```python
from build123d import *

# Parameters (mm, degrees)
F0_W     = 38.1
F0_H     = 50.8
F1_DEPTH = 18.288
F2_SIZE  = 5.08


with BuildPart() as f1:
    # F0 (on Top) → F1 (new body)
    with BuildSketch(Plane.XY):
        with Locations((32.766, -53.848)):
            Rectangle(F0_W, F0_H)
        Polygon((65.532, -18.288), (0, -18.288), (0, 0), (-1.016, 0), (-4.572, -18.288), (-4.572, -28.448), (13.716, -28.448), (51.816, -28.448), (70.104, -28.448), (70.104, -18.288), (66.548, 0), (65.532, 0), align=None)
    extrude(amount=F1_DEPTH)

    # F2
    f2_edges = [f1.edges().sort_by_distance(p)[0] for p in [
        (13.716, -53.848, 18.288),
        (51.816, -53.848, 18.288),
        (51.816, -53.848, 0),
        (13.716, -53.848, 0),
        (-4.572, -28.448, 9.144),
        (70.104, -28.448, 9.144),
    ]]
    chamfer(f2_edges, length=F2_SIZE)


solid = f1.part
```
The listing builds one solid part. Answer for the finished solid, in the listing's coordinates (mm). A direction names the side the tool comes from. Give positions to 0.01 mm unless a question says otherwise; leave off trailing zeros. Order: outer loops, then holes, each group sorted by start corner. A loop starts at its lowest first (then second) coordinate and runs counter-clockwise, first axis right, second up. Notation, with made-up numbers: (-35, -2) -> (2, -2) arc R11 cw to (2, 7) -> close; hole circle Ø10 at (15.25, 78.5). An arc over 180 degrees is marked (long way). One line per item, written item: value.
1) Find section C-C, the plane y = -11.5. Determine the outline of the cut face in (x, z), plus the area to 3 significant figures.
Reported:
outline: (-3.25, 0) -> (0, 0) -> (0, 18.29) -> (-3.25, 18.29) -> close; (65.53, 0) -> (68.78, 0) -> (68.78, 18.29) -> (65.53, 18.29) -> close
area: 119 mm^2
2) Find section A-A, the plane y = -53. Determine the outline of the cut face in (x, z), plus the area to 3 significant figures.
Reported:
outline: (13.72, 5.08) -> (18.8, 0) -> (46.74, 0) -> (51.82, 5.08) -> (51.82, 13.21) -> (46.74, 18.29) -> (18.8, 18.29) -> (13.72, 13.21) -> close
area: 645 mm^2
3) A tool of negligible diameter and unlimited length cuts with its end or side. For faces 4 (the flat face through (49.24, -54.204, 15.784)), 5 (the flat face through (33, -18.288, 9)), 6 (the flat face through (49.24, -54.204, 2.504)), from which of +Z, -Z, +X, -X, +Y, -Y can it reach the whole face along a straight path? Write none if from no direction.
Reported:
face 4: +Z, +X, -Y
face 5: +Z, -Z, +Y
face 6: -Z, +X, -Y
4) Find section D-D, the plane x = 10. Determine the outline of the cut face in (y, z).
Reported:
outline: (-28.45, 0) -> (-18.29, 0) -> (-18.29, 18.29) -> (-28.45, 18.29) -> close
5) Determine the mould class of faces 1 (the flat face through (65.532, -9, 9)), 2 (the flat face through (51.816, -54, 9)), 3 (the flat face through (33, -37, 18.288)) for opening direction X: pulls with the +X half, pulls with the -X half, needs draft (parallel to the pull), parting line crosses it, or undercut.
Reported:
face 1: undercut
face 2: pulls with the +X half
face 3: needs draft
6) Find the intervals of material crossed by line 1 (Y direction, x = 14.5, z = 14.5); line 2 (X direction, y = -59, z = 11); line 3 (Y direction, x = 34.5, z = 14.5), in increasing order.
Reported:
line 1: y = -28.45 to -18.29
line 2: x = 13.72 to 51.82
line 3: y = -79.25 to -18.29
7) Flat-ended cylindrical pins translate along their axes: P1, Ø5.5, axis at x = 8, z = 7.5, coming from the -Y side; P2, Ø6.5, axis at y = -41.5, z = 7.5, coming from the -X side; P3, Ø1.5, axis at x = 42.5, z = 7, coming from the +Y side; P4, Ø10, axis at x = 24.5, y = -11.5, coming from the -Z side. Find the tip coordinate at first contact, or state that the pin passes through.
Reported:
P1: stops at y = -28.45
P2: stops at x = 13.72
P3: stops at y = -18.29
P4: passes through
8) Find section B-B, the plane z = 8.5. Determine the outline of the cut face in (x, y), plus the area to 3 significant figures.
Reported:
outline: (-4.57, -23.37) -> (0.51, -28.45) -> (13.72, -28.45) -> (13.72, -79.25) -> (51.82, -79.25) -> (51.82, -28.45) -> (65.02, -28.45) -> (70.1, -23.37) -> (70.1, -18.29) -> (66.55, 0) -> (65.53, 0) -> (65.53, -18.29) -> (0, -18.29) -> (0, 0) -> (-1.02, 0) -> (-4.57, -18.29) -> close
area: 2,770 mm^2
